Could you check a few things on this model? Use its own coordinates, in mm. A direction names the side the tool comes from. Round coordinates to 2 decimals unless told otherwise and drop trailing zeros. Loops run counter-clockwise (first coordinate to the right, second up) from the corner with the lowest first, then second, coordinate; pieces in that order, holes last. Notation, with made-up numbers: (83.25, 51.5) - (88.25, 51.5) arc R27 ccw to (88.25, 74.5) - close; hole circle Ø7 at (19, 28). An arc over 180 degrees is marked (long way). Answer as CSV lines item,"result". Start each with the question number.
1) We'd pull the mould along Z, two halves only. Please class faces 1 (the face through (-7.993, -50.026, -79.692)), 2 (the face through (7, -25.4, 11)), 3 (the face through (-48.651, -12.522, -27.715)), 4 (the face through (-12, -101.328, -5)): pulls with the +Z half, pulls with the -Z half, needs draft (parallel to the pull), parting line crosses it, or undercut.
2) Suppose I cut it at B-B, the plane y = -36. Write out the boundary of the cut face in (x, z), then the cut area to 3 significant figures.
3) Which directions (+Z, -Z, +X, -X, +Y, -Y) give clear straight access to the entire face, cutting with the end or side of a thin tool? Please do faces 5 (the face through (-2.948, -12.522, -74.257)), 6 (the face through (-18, 0, -14)).
4) Please list where these lines run through material, in increasing order: line 1 along X through (y, z) = (-24, -41.5); line 2 along Y through (x, z) = (-63, 6); line 3 along X through (y, z) = (-11, -27.5).
5) Suppose I cut it at A-A, the plane y = -19. Write out the boundary of the cut face in (x, z).
6) I'm going to push flat-ended pins straight in: pin 1 Ø10 at (x, z) = (9.5, 7.5) entering from +Y; pin 2 Ø3 at (x, y) = (-63.5, -37) entering from +Z; pin 3 Ø5 at (y, z) = (-16, 29.5) entering from +X; pin 4 Ø3 at (y, z) = (-84.5, 36) entering from +X. Where does each tip first touch, or does it pass through?
```python
from build123d import *

# Parameters (mm, degrees)
F1_DEPTH = 101.3275142759
F2_R     = 5.08
F3_R     = 5.08
F4_R     = 33.6683926693
F5_DEPTH = 25.4


with BuildPart() as f1:
    # F0 (on Front) → F1 (new body)
    with BuildSketch(Plane.XZ):
        with BuildLine():
            Line((32.1733355522, 64.3209666014), (-61.8066638708, 57.9346120358))
            ThreePointArc((-61.8066638708, 57.9346120358), (-5.2566823209, -79.5545167495), (32.1733355522, 64.3209666014))
        make_face()
    extrude(amount=F1_DEPTH)

    # F2
    f2_edges = [f1.edges().sort_by_distance(p)[0] for p in [
        (-5.256682, -101.327514, -79.554517),
    ]]
    fillet(f2_edges, radius=F2_R)

    # F3
    f3_edges = [f1.edges().sort_by_distance(p)[0] for p in [
        (-5.256682, 0, -79.554517),
    ]]
    fillet(f3_edges, radius=F3_R)

    # F4 (on face) → F5 (cut)
    with BuildSketch(Plane(origin=(0, 0, 0), x_dir=(-1, 0, 0), z_dir=(0, 1, 0))):
        with BuildLine():
            ThreePointArc((-23.146174833, 63.7075313021), (5.6010963761, -74.4862054964), (52.7795031516, 58.548047335))
            Line((52.7795031516, 58.548047335), (-23.146174833, 63.7075313021))
        make_face()
        with Locations((17.5497084856, -14.8196211085)):
            Circle(F4_R, mode=Mode.SUBTRACT)
    extrude(amount=-F5_DEPTH, mode=Mode.SUBTRACT)


solid = f1.part
```
Filled sheet:
1,face 1,"parting line crosses it"
1,face 2,"undercut"
1,face 3,"undercut"
1,face 4,"needs draft"
2,outline,"(-61.81, 57.93) arc R78.37 ccw (long way) to (32.17, 64.32) - close"
2,area,"18,300 mm²"
3,face 5,"+Y"
3,face 6,"+Z, -Z, +X, -X, +Y"
4,line 1,"-77.88 to -71.89, -38.09 to 2.99, 50.75 to 56.74"
4,line 2,"-101.33 to -25.4"
4,line 3,"-84.45 to -79.04, -48.74 to 13.64, 57.9 to 63.31"
5,outline,"(-61.81, 57.93) arc R78.37 ccw (long way) to (32.17, 64.32) - (23.15, 63.71) arc R73.29 cw (long way) to (-52.78, 58.55) - close; circle Ø67.34 at (-17.55, -14.82)"
6,pin 1,"y = 0"
6,pin 2,"z = 57.77"
6,pin 3,"x = 62.49"
6,pin 4,"x = 59.11"
